Can you work these out from the model? Positions are in its coordinate system, mm. Round coordinates to 2 decimals unless told otherwise and drop trailing zeros. Loops run counter-clockwise (first coordinate to the right, second up) from the corner with the lowest first, then second, coordinate; pieces in that order, holes last. Notation, with made-up numbers: (-21.75, 80.5) -> (-5.75, 80.5) arc R21 cw to (-5.75, 115.5) -> close; hole circle Ø10 at (-36.5, 9). An arc over 180 degrees is marked (long way). Answer as a JSON object with one key per item and string values.
```python
from build123d import *

# Parameters (mm, degrees)
SKETCH1_W                             = 12.7
SKETCH1_H                             = 12.7
BOSS_EXTRUDE1_DEPTH                   = 101.6
F_1_4_20_TAPPED_HOLE1_D               = 5.1054
F_1_4_20_TAPPED_HOLE1_DEPTH           = 16.51
F_1_4_20_TAPPED_HOLE1_TIP             = 1.533816902
F_1_4_20_TAPPED_HOLE1_ON_FACE_2_D     = 5.1054
F_1_4_20_TAPPED_HOLE1_ON_FACE_2_DEPTH = 16.51
F_1_4_20_TAPPED_HOLE1_ON_FACE_2_TIP   = 1.533816902
F_1_4_20_TAPPED_HOLE2_D               = 5.1054
F_1_4_20_TAPPED_HOLE2_DEPTH           = 16.51
F_1_4_20_TAPPED_HOLE2_TIP             = 1.533816902
F_1_4_20_TAPPED_HOLE3_D               = 5.1054
F_1_4_20_TAPPED_HOLE3_DEPTH           = 16.51
F_1_4_20_TAPPED_HOLE3_TIP             = 1.533816902


with BuildPart() as part:
    # Sketch1 → Boss-Extrude1 (new body)
    with BuildSketch(Plane(origin=(0, 0, 0), x_dir=(1, 0, 0), z_dir=(0, 1, 0))):
        with Locations((6.35, -6.35)):
            Rectangle(SKETCH1_W, SKETCH1_H)
    extrude(amount=BOSS_EXTRUDE1_DEPTH)

    # 1/4-20 Tapped Hole1
    with Locations(Plane(origin=(6.35, 0, 6.35), x_dir=(0, 0, -1), z_dir=(0, -1, 0))):
        with Locations((0, 0)):
            Hole(F_1_4_20_TAPPED_HOLE1_D / 2, depth=F_1_4_20_TAPPED_HOLE1_DEPTH)
            with Locations((0, 0, -(F_1_4_20_TAPPED_HOLE1_DEPTH + F_1_4_20_TAPPED_HOLE1_TIP / 2))):  # 118° drill point
                Cone(0, F_1_4_20_TAPPED_HOLE1_D / 2, F_1_4_20_TAPPED_HOLE1_TIP, mode=Mode.SUBTRACT)

    # 1/4-20 Tapped Hole1 on face 2
    with Locations(Plane(origin=(6.35, 101.6, 6.35), x_dir=(0, 0, 1), z_dir=(0, 1, 0))):
        with Locations((0, 0)):
            Hole(F_1_4_20_TAPPED_HOLE1_ON_FACE_2_D / 2, depth=F_1_4_20_TAPPED_HOLE1_ON_FACE_2_DEPTH)
            with Locations((0, 0, -(F_1_4_20_TAPPED_HOLE1_ON_FACE_2_DEPTH + F_1_4_20_TAPPED_HOLE1_ON_FACE_2_TIP / 2))):  # 118° drill point
                Cone(0, F_1_4_20_TAPPED_HOLE1_ON_FACE_2_D / 2, F_1_4_20_TAPPED_HOLE1_ON_FACE_2_TIP, mode=Mode.SUBTRACT)

    # 1/4-20 Tapped Hole2
    with Locations(Plane(origin=(6.35, 76.2, 0), x_dir=(-1, 0, 0), z_dir=(0, 0, -1))):
        with Locations((0, 0), (0, -35.56)):
            Hole(F_1_4_20_TAPPED_HOLE2_D / 2, depth=F_1_4_20_TAPPED_HOLE2_DEPTH)
            with Locations((0, 0, -(F_1_4_20_TAPPED_HOLE2_DEPTH + F_1_4_20_TAPPED_HOLE2_TIP / 2))):  # 118° drill point
                Cone(0, F_1_4_20_TAPPED_HOLE2_D / 2, F_1_4_20_TAPPED_HOLE2_TIP, mode=Mode.SUBTRACT)

    # 1/4-20 Tapped Hole3
    with Locations(Plane(origin=(12.7, 25.4, 6.35), x_dir=(0, 0, 1), z_dir=(1, 0, 0))):
        with Locations((0, 0), (0, -38.1)):
            Hole(F_1_4_20_TAPPED_HOLE3_D / 2, depth=F_1_4_20_TAPPED_HOLE3_DEPTH)
            with Locations((0, 0, -(F_1_4_20_TAPPED_HOLE3_DEPTH + F_1_4_20_TAPPED_HOLE3_TIP / 2))):  # 118° drill point
                Cone(0, F_1_4_20_TAPPED_HOLE3_D / 2, F_1_4_20_TAPPED_HOLE3_TIP, mode=Mode.SUBTRACT)


solid = part.part
```
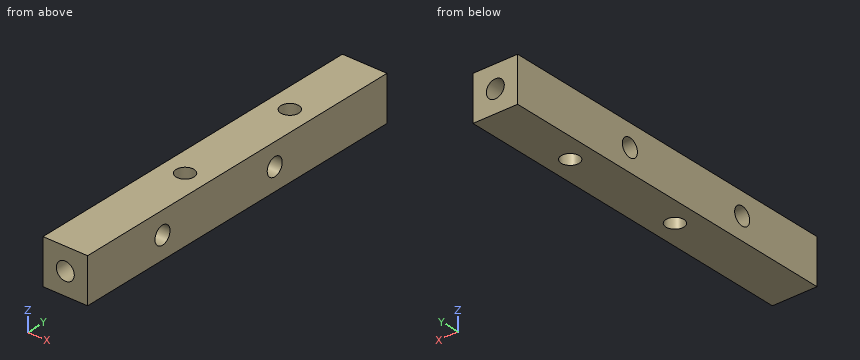
Q1. I want a section at B-B, the plane z = 1. Write out the boundary of the cut face in (x, y).
Determined:
{"outline": "(0, 0) -> (12.7, 0) -> (12.7, 101.6) -> (0, 101.6) -> close; hole circle Ø5.11 at (6.35, 40.64); hole circle Ø5.11 at (6.35, 76.2)"}
Q2. I'm going to push a flat-ended pin straight in: pin 1 (1.5 mm diameter, centred on y = 19, z = 10.5, fed in from -X). Where does the tip first touch, or does it pass through?
Determined:
{"pin 1": "x = 0"}
Q3. I want a section at D-D, the plane x = 9.75. Write out the boundary of the cut face in (y, z), then the cut area to 3 significant figures.
Determined:
{"outline": "(0, 0) -> (101.6, 0) -> (101.6, 12.7) -> (0, 12.7) -> close; hole circle Ø5.11 at (25.4, 6.35); hole circle Ø5.11 at (63.5, 6.35)", "area": "1,250 mm²"}
Q4. If I drill on L1, parallel to Y at x = 6.35, z = 10.25; L2, parallel to X at y = 5.25, z = 6.35, over which ranges is the centre line in solid material (lowest first)? Write a range as [from, to].
Determined:
{"L1": "[0, 38.09], [43.19, 73.65], [78.75, 101.6]", "L2": "[0, 3.8], [8.9, 12.7]"}
Q5. I want a section at C-C, the plane y = 14. Write out the boundary of the cut face in (x, z).
Determined:
{"outline": "(0, 0) -> (12.7, 0) -> (12.7, 12.7) -> (0, 12.7) -> close; hole circle Ø5.11 at (6.35, 6.35)"}
Q6. I want a section at A-A, the plane y = 25.4. Write out the boundary of the cut face in (x, z), then the cut area to 3 significant figures.
Determined:
{"outline": "(0, 0) -> (12.7, 0) -> (12.7, 3.8) -> (0, 3.8) -> close; (0, 8.9) -> (12.7, 8.9) -> (12.7, 12.7) -> (0, 12.7) -> close", "area": "96.5 mm²"}
